Could you check a few things on this model? Use its own coordinates, in mm. Coordinates: 2 decimals unless noted, no trailing zeros. Loops run counter-clockwise (first coordinate to the right, second up) from the corner with the lowest first, then second, coordinate; pieces in that order, holes last. Notation, with made-up numbers: M 6.5,-7.5 L 21.5,-7.5 A29 cw 21.5,13.5 Z; hole C 14.25,41.5 d1. An arc over 180 degrees is marked long. Write each question's results on one line, items separated by ' | '.
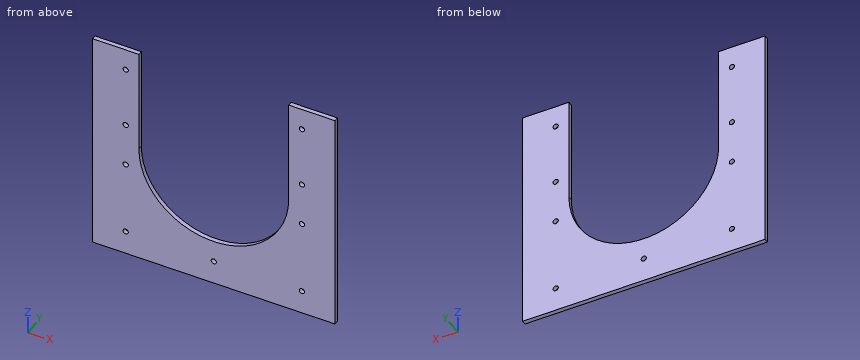
```python
from build123d import *

# Parameters (mm, degrees)
SKETCH005_R      = 6
EXTRUDE004_DEPTH = 1000
EXTRUDE003_DEPTH = 1000
SKETCH003_W      = 550
SKETCH003_H      = 10
EXTRUDE002_DEPTH = 515


with BuildPart() as extrude004:
    # Sketch005 → Extrude004 (new body)
    with BuildSketch(Plane.XZ.offset(2500)):
        with Locations((-200, 1730)):
            Circle(SKETCH005_R)
        with Locations((-200, 1870)):
            Circle(SKETCH005_R)
        with Locations((200, 1870)):
            Circle(SKETCH005_R)
        with Locations((200, 1730)):
            Circle(SKETCH005_R)
        with Locations((-200, 1630)):
            Circle(SKETCH005_R)
        with Locations((-200, 1460)):
            Circle(SKETCH005_R)
        with Locations((200, 1630)):
            Circle(SKETCH005_R)
        with Locations((200, 1460)):
            Circle(SKETCH005_R)
        with Locations((0, 1460)):
            Circle(SKETCH005_R)
    extrude(amount=-EXTRUDE004_DEPTH)


with BuildPart() as extrude003:
    # Sketch004 → Extrude003 (new body)
    with BuildSketch(Plane.XZ.offset(2500)):
        with BuildLine():
            Line((-170, 1920), (-170, 1680))
            ThreePointArc((-170, 1680), (-4.8e-05, 1510), (170, 1679.999905))
            Line((170, 1679.999905), (170, 1920))
            Line((170, 1920), (-170, 1920))
        make_face()
    extrude(amount=-EXTRUDE003_DEPTH)


with BuildPart() as cut002:
    # Sketch003 → Extrude002 (new body)
    with BuildSketch(Plane.XY.offset(1405)):
        with Locations((0, -1670.580576)):
            Rectangle(SKETCH003_W, SKETCH003_H)
    extrude(amount=EXTRUDE002_DEPTH)

    # Cut001: cut Extrude003
    add(extrude003.part, mode=Mode.SUBTRACT)

    # Cut002: cut Extrude004
    add(extrude004.part, mode=Mode.SUBTRACT)


solid = cut002.part
```
(1) Please list where these lines run through material, in increasing order: probe 1 along X at (y, z) = (-1671.25, 1460); probe 2 along Z at (x, y) = (200, -1671); probe 3 along X at (y, z) = (-1672, 1730). Write a range as from..to.
Reported:
probe 1: x = -275..-206, -194..-6, 6..194, 206..275 | probe 2: z = 1405..1454, 1466..1624, 1636..1724, 1736..1864, 1876..1920 | probe 3: x = -275..-206, -194..-170, 170..194, 206..275
(2) Will these pins go through, and if not, where does the flat tip stop? P1, Ø5, axis at x = 72, y = -1669, coming from the +Z side; P2, Ø1.5, axis at x = 9, y = -1672, coming from the +Z side.
Reported:
P1: stops at z = 1527.19 | P2: stops at z = 1510.28
(3) Imagine slicing it at A-A, the plane z = 1790.5. List the corners of the cut face in (x, y) for me, and give its area (3 significant figures).
Reported:
outline: M -275,-1675.58 L -170,-1675.58 L -170,-1665.58 L -275,-1665.58 Z; M 170,-1675.58 L 275,-1675.58 L 275,-1665.58 L 170,-1665.58 Z | area: 2,100 mm2
(4) Imagine slicing it at D-D, the plane x = -51.5. List the corners of the cut face in (y, z) for me, and give its area (3 significant figures).
Reported:
outline: M -1675.58,1405 L -1665.58,1405 L -1665.58,1517.99 L -1675.58,1517.99 Z | area: 1,130 mm2
(5) Imagine slicing it at C-C, the plane x = 56. List the corners of the cut face in (y, z) for me, and give its area (3 significant figures).
Reported:
outline: M -1675.58,1405 L -1665.58,1405 L -1665.58,1519.49 L -1675.58,1519.49 Z | area: 1,140 mm2
(6) Imagine slicing it at B-B, the plane y = -1669.5. State how many separate pieces and enclosed holes the cut face has, and give its area (3 significant figures).
Reported:
separate pieces: 1 | enclosed holes: 9 | area: 155,000 mm2
